Autodesk Inventor part; units mm, degrees
ref_plane "YZ Plane" through (0, 0, 0) normal (1, 0, 0) x (0, 1, 0)
ref_plane "XZ Plane" through (0, 0, 0) normal (0, 1, 0) x (-1, 0, 0)
ref_plane "XY Plane" through (0, 0, 0) normal (0, 0, 1) x (1, 0, 0)
sketch "Sketch1" plane through (0, 0, 0) normal (0, 0, 1) x (1, 0, 0)
  circle A0 centre (0, 0) radius 4
  circle A1 centre (0, 0) radius 12.5
  circle A2 centre (0, 150) radius 4
  circle A3 centre (0, 150) radius 12.5
  line L0 (-12.5, 150) -> (-12.5, 0)
  line L1 (12.5, 150) -> (12.5, 0)
  dimension "d0" = 8
  dimension "d1" = 25
  dimension "d2" = 8
  dimension "d3" = 25
  dimension "d4" = 150
  dimension "d5" = 0
extrude "Extrusion1" add sketch "Sketch1" along normal blind 5
equation "\"d2\" = d0"
equation "\"d3\" = d1"
properties part number "cięgno silnika platformy"
Model file for the job. Use its own axes, mm. Give positions to 0.01 mm unless a question says otherwise; leave off trailing zeros. Loops run counter-clockwise (first coordinate to the right, second up) from the corner with the lowest first, then second, coordinate; pieces in that order, holes last. Notation, with made-up numbers: (-38, 81) - (-28, 81) arc R18 cw to (-28, 89) - close; hole circle Ø9 at (40, 76.25). An arc over 180 degrees is marked (long way). One line per item, written item: value. Start each with the question number.
1. Slice it at B-B (z = 2.8). List the corners of the cut face in (x, y), plus the area to 3 significant figures.
2. Slice it at C-C (x = -6.25). List the corners of the cut face in (y, z), plus the area to 3 significant figures.
3. Pull direction Y, two halves, no side cores. Call faces 1 (the cylindrical face through (-0.867, 3.905, 2.465)), 2 (the flat face through (0, 76, 5)), 3 (the cylindrical face through (0.275, -12.497, 2.465)): pulls with the +Y half, pulls with the -Y half, needs draft (parallel to the pull), parting line crosses it, or undercut.
4. Slice it at D-D (x = 10.5). List the corners of the cut face in (y, z), plus the area to 3 significant figures.
5. Pin check, flat tips, straight feed: pin 1 (1 mm diameter, centred on x = -6, z = 3.5, fed in from -Y) (3 decimals); pin 2 (7 mm diameter, centred on x = 0, y = 0, fed in from +Z); pin 3 (2 mm diameter, centred on x = -4, z = 1, fed in from -Y). Stop position of each tip, or through.
6. Probe L1, parallel to Y at x = 0, z = 3.95; L2, parallel to Y at x = -1.5, z = 3.2; L3, parallel to X at y = -0.5, z = 1.15. List the from-to ranges inside material, lowest first. Write a range as from..to.
7. Slice it at A-A (x = 0). List the corners of the cut face in (y, z).
Solution:
1. outline: (-12.5, 0) arc R12.5 ccw to (12.5, 0) - (12.5, 150) arc R12.5 ccw to (-12.5, 150) - close; hole circle Ø8 at (0, 0); hole circle Ø8 at (0, 150)
1. area: 4,140 mm^2
2. outline: (-10.83, 0) - (160.83, 0) - (160.83, 5) - (-10.83, 5) - close
2. area: 858 mm^2
3. face 1: undercut
3. face 2: needs draft
3. face 3: pulls with the -Y half
4. outline: (-6.78, 0) - (156.78, 0) - (156.78, 5) - (-6.78, 5) - close
4. area: 818 mm^2
5. pin 1: stops at y = -11.225
5. pin 2: passes through
5. pin 3: stops at y = -12.13
6. L1: y = -12.5..-4, 4..146, 154..162.5
6. L2: y = -12.41..-3.71, 3.71..146.29, 153.71..162.41
6. L3: x = -12.49..-3.97, 3.97..12.49
7. outline: (-12.5, 0) - (-4, 0) - (-4, 5) - (-12.5, 5) - close; (4, 0) - (146, 0) - (146, 5) - (4, 5) - close; (154, 0) - (162.5, 0) - (162.5, 5) - (154, 5) - close
